Check sheet for the modelled part. Datum: model origin and axes. Units: mm. A direction names the side the tool comes from. Give positions to 0.01 mm unless a question says otherwise; leave off trailing zeros. Order: outer loops, then holes, each group sorted by start corner. A loop starts at its lowest first (then second) coordinate and runs counter-clockwise, first axis right, second up. Notation, with made-up numbers: (-21, 38) - (20, 38) arc R30 cw to (20, 61) - close; hole circle Ø5 at (-16, -19.5). An arc over 180 degrees is marked (long way). Answer in a Markdown table with one row per item.
from build123d import *

# Parameters (mm, degrees)
SCALE1_SCALE = 0.6


with BuildPart() as part:
    # Sketch1 → Revolve1 (revolve)
    with BuildSketch(Plane(origin=(0, 0, 0), x_dir=(0, 0, -1), z_dir=(1, 0, 0)), mode=Mode.PRIVATE) as revolve1_sk:
        Polygon((0, -8.0645), (28.448, -8.0645), (28.448, 0), (31.75, 0), (31.75, -10.033), (26.1112, -11.811), (26.1112, -9.7282), (21.7932, -9.7282), (21.7932, -13.335), (9.9568, -13.335), (9.9568, -9.7282), (5.6388, -9.7282), (5.6388, -11.811), (0, -10.033), align=None)
    revolve(revolve1_sk.sketch.rotate(Axis((0, 0, 0), (0, 0, -1)), 270), axis=Axis((0, 0, 0), (0, 0, -1)))


with BuildPart() as part_1:
    # Scale1: scaled about (0, 0, -17.137127413)
    add(part.part.scale(SCALE1_SCALE).moved(Location((0, 0, -6.854850965))))


solid = part_1.part
(1) Gauge pin test, flat ends, axial feed: P1, Ø4, axis at x = 3.5, z = -12, coming from the +Y side; P2, Ø3, axis at y = -0.5, z = -11, coming from the -X side; P3, Ø5, axis at x = 1.5, y = -0.5, coming from the +Z side; P4, Ø8, axis at x = 0.5, y = -1, coming from the +Z side. Record the tip position at first contact, or that the pin passes through.
Geometry says:
| item | result |
|---|---|
| P1 | y = 7.82 |
| P2 | x = -7.09 |
| P3 | z = -23.92 |
| P4 | z = -6.85 |
(2) Mould release check, pull along X, two halves, no side actions. Record for faces 4 (the cylindrical face through (5.57, -1.75, -11.52)), 5 (the cylindrical face through (-3.84, 2.944, -15.509)), 6 (the flat face through (1, 6, -12.829)): pulls with the +X half, pulls with the -X half, needs draft (parallel to the pull), parting line crosses it, or undercut.
Geometry says:
| item | result |
|---|---|
| face 4 | parting line crosses it |
| face 5 | undercut |
| face 6 | needs draft |
(3) Access from +Z, -Z, +X, -X, +Y, -Y to the whole of each face (thin tool, end or side, straight path). Record for faces 1 (the flat face through (0, -5, -6.855)), 2 (the flat face through (0, 0, -23.924)), 3 (the flat face through (-1, 6, -19.931)).
Geometry says:
| item | result |
|---|---|
| face 1 | +Z, +X, -X, +Y, -Y |
| face 2 | +Z |
| face 3 | none |
(4) Cross-section at A-A, the plane x = 0. Record the cut outline in (y, z), then the cut area to 3 significant figures.
Geometry says:
| item | result |
|---|---|
| outline | (-8, -19.93) - (-5.84, -19.93) - (-5.84, -22.52) - (-7.09, -22.52) - (-6.02, -25.9) - (6.02, -25.9) - (7.09, -22.52) - (5.84, -22.52) - (5.84, -19.93) - (8, -19.93) - (8, -12.83) - (5.84, -12.83) - (5.84, -10.24) - (7.09, -10.24) - (6.02, -6.85) - (4.84, -6.85) - (4.84, -23.92) - (-4.84, -23.92) - (-4.84, -6.85) - (-6.02, -6.85) - (-7.09, -10.24) - (-5.84, -10.24) - (-5.84, -12.83) - (-8, -12.83) - close |
| area | 97.6 mm² |
(5) Cross-section at C-C, the plane z = -21. Record the cut outline in (x, y).
Geometry says:
| item | result |
|---|---|
| outline | circle Ø11.67 at (0, 0); hole circle Ø9.68 at (0, 0) |
(6) Cross-section at D-D, the plane z = -14.75. Record the cut outline in (x, y), then the cut area to 3 significant figures.
Geometry says:
| item | result |
|---|---|
| outline | circle Ø16 at (0, 0); hole circle Ø9.68 at (0, 0) |
| area | 128 mm² |
(7) Thickness scan on L1, parallel to Z at x = 5.75, y = 1.5; L2, parallel to Y at x = 0, z = -14.75; L3, parallel to Y at x = 0, z = -11.25. Record the ranges inside material, lowest first.
Geometry says:
| item | result |
|---|---|
| L1 | -25.9 to -22.52, -19.93 to -12.83, -10.24 to -6.85 |
| L2 | -8 to -4.84, 4.84 to 8 |
| L3 | -5.84 to -4.84, 4.84 to 5.84 |
